Can you work these out from the model? Positions are in its coordinate system, mm. Coordinates: 2 decimals unless noted, no trailing zeros. Order: outer loops, then holes, each group sorted by start corner. A loop starts at its lowest first (then second) coordinate and runs counter-clockwise, first axis right, second up. Notation, with made-up numbers: (58.5, 17) -> (77.5, 17) arc R22 ccw to (77.5, 48) -> close; hole circle Ø2 at (47, -35.5). An arc over 180 degrees is marked (long way). Answer as CSV lines item,"result".
from build123d import *

# Parameters (mm, degrees)
BOSS_EXTRUDE1_DEPTH = 6
SKETCH2_W           = 31.8008
SKETCH2_H           = 5.588
SKETCH2_H_2         = 2.7432
TABS_DEPTH          = 6
FILLET2_R           = 6.35
FILLET3_R           = 6.35
SKETCH5_W           = 6.35
SKETCH5_H           = 25.4
TAB_CUT_OUTS_DEPTH  = 6


with BuildPart() as part:
    # Sketch1 → Boss-Extrude1 (new body)
    with BuildSketch(Plane(origin=(0, 0, 0), x_dir=(1, 0, 0), z_dir=(0, 1, 0))):
        Polygon((-190.5, -76.2), (190.5, -76.2), (133.35, 76.2), (-133.35, 76.2), align=None)
    extrude(amount=BOSS_EXTRUDE1_DEPTH)

    # Sketch2 → Tabs (add)
    with BuildSketch(Plane(origin=(0, 6, 0), x_dir=(1, 0, 0), z_dir=(0, 1, 0))):
        with Locations((95.25, 78.994)):
            Rectangle(SKETCH2_W, SKETCH2_H)
        with Locations((-31.75, 78.994)):
            Rectangle(SKETCH2_W, SKETCH2_H)
        with Locations((-95.25, 78.994)):
            Rectangle(SKETCH2_W, SKETCH2_H)
        with Locations((31.75, 78.994)):
            Rectangle(SKETCH2_W, SKETCH2_H)
        with Locations((53.975, -77.5716)):
            Rectangle(SKETCH2_W, SKETCH2_H_2)
        with Locations((-53.975, -77.5716)):
            Rectangle(SKETCH2_W, SKETCH2_H_2)
        with Locations((-158.75, -77.5716)):
            Rectangle(SKETCH2_W, SKETCH2_H_2)
        with Locations((158.75, -77.5716)):
            Rectangle(SKETCH2_W, SKETCH2_H_2)
    extrude(amount=-TABS_DEPTH)

    # Fillet2
    fillet2_edges = [part.edges().sort_by_distance(p)[0] for p in [
        (190.5, 3, 76.2),
        (-190.5, 3, 76.2),
    ]]
    fillet(fillet2_edges, radius=FILLET2_R)

    # Fillet3
    fillet3_edges = [part.edges().sort_by_distance(p)[0] for p in [
        (-133.35, 3, -76.2),
        (133.35, 3, -76.2),
    ]]
    fillet(fillet3_edges, radius=FILLET3_R)

    # Sketch5 → Tab Cut Outs (cut)
    with BuildSketch(Plane(origin=(0, 6, 0), x_dir=(1, 0, 0), z_dir=(0, 1, 0))):
        with Locations((127, -38.1)):
            Rectangle(SKETCH5_W, SKETCH5_H)
        with Locations((127, 38.1)):
            Rectangle(SKETCH5_W, SKETCH5_H)
        with Locations((127, 0)):
            Rectangle(SKETCH5_W, SKETCH5_H)
    tab_cut_outs = extrude(amount=-TAB_CUT_OUTS_DEPTH, mode=Mode.SUBTRACT)

    # Mirror1: Tab Cut Outs across plane
    add(tab_cut_outs.mirror(Plane.ZY), mode=Mode.SUBTRACT)


solid = part.part
Q1. Imagine slicing it at C-C (x = 103.5). List the corners of the cut face in (y, z) for me.
Solution:
outline,"(0, -81.79) -> (6, -81.79) -> (6, 76.2) -> (0, 76.2) -> close"
Q2. For P1, Ø1.8, axis at x = -126, y = 1.5, coming from the +Z side; P2, Ø3, axis at y = 4.5, z = 78.5, coming from the -X side; P3, Ø3, axis at x = -60.5, z = 26, coming from the -Y side; P4, Ø1.7, axis at y = 4, z = -80, coming from the +X side, each with a flat end and sliding along its axis, tell me the tip position at first contact or that it passes through.
Solution:
P1,"z = 76.2"
P2,"x = -174.65"
P3,"y = 0"
P4,"x = 111.15"
Q3. If I drill on line 1 (X direction, y = 1.3, z = 49) (3 decimals); line 2 (X direction, y = 4.75, z = -10) (3 decimals); line 3 (Z direction, x = 23.5, y = 2), over which ranges is the centre line in solid material (lowest first)?
Solution:
line 1,"-180.3 to -130.175, -123.825 to 123.825, 130.175 to 180.3"
line 2,"-158.175 to -130.175, -123.825 to 123.825, 130.175 to 158.175"
line 3,"-81.79 to 76.2"
Q4. Imagine slicing it at D-D (z = -67). List the corners of the cut face in (x, y) for me, and give its area (3 significant figures).
Solution:
outline,"(-136.8, 0) -> (136.8, 0) -> (136.8, 6) -> (-136.8, 6) -> close"
area,"1,640 mm2"
Q5. Imagine slicing it at B-B (y = 1.9). Give the number of separate pieces and of enclosed holes in the cut face, and give its area (3 significant figures).
Solution:
separate pieces,"1"
enclosed holes,"6"
area,"49,400 mm2"
Q6. Imagine slicing it at A-A (z = -0.5). List the corners of the cut face in (x, y) for me (1 decimal), and give its area (3 significant figures).
Solution:
outline,"(-161.7, 0) -> (-130.2, 0) -> (-130.2, 6) -> (-161.7, 6) -> close; (-123.8, 0) -> (123.8, 0) -> (123.8, 6) -> (-123.8, 6) -> close; (130.2, 0) -> (161.7, 0) -> (161.7, 6) -> (130.2, 6) -> close"
area,"1,860 mm2"
